Read the model definition and answer for the solid it produces. Units are mm, in the model's axes. A direction names the side the tool comes from. Round coordinates to 2 decimals unless told otherwise and drop trailing zeros. Write each loop counter-clockwise with the first axis right and the second up, starting at its lowest first coordinate (ties: lowest second). Pieces come first, ordered by that corner, then holes.
from build123d import *

# Parameters (mm, degrees)
BOSS_EXTRUDE1_DEPTH = 46.736
SKETCH3_W           = 38.481
SKETCH3_H           = 38.481
BOSS_EXTRUDE2_DEPTH = 17.526
SKETCH_D_R          = 7.9375
BOSS_EXTRUDE3_DEPTH = 38.1
CUT_EXTRUDE1_DEPTH  = 35.56
FILLET1_R           = 6.35
FILLET2_R           = 1.27
KEYWAY_START        = 5.1943
KEYWAY_DEPTH        = 33.9057
CHAMFER1_SIZE       = 0.381
SKETCH7_R           = 7.9375
CUT_EXTRUDE3_DEPTH  = 103.362


with BuildPart() as part:
    # L,M → Boss-Extrude1 (new body)
    with BuildSketch(Plane.XY):
        Polygon((-44.45, 31.75), (44.45, 31.75), (44.45, 90.644463274), (36.576, 98.518463274), (36.576, 130.081536726), (14.257536726, 152.4), (-14.257536726, 152.4), (-36.576, 130.081536726), (-36.576, 98.518463274), (-44.45, 90.644463274), align=None)
    extrude(amount=BOSS_EXTRUDE1_DEPTH)

    # Sketch3 → Boss-Extrude2 (add)
    with BuildSketch(Plane.XY.offset(46.736)):
        with Locations((0, 114.3)):
            Rectangle(SKETCH3_W, SKETCH3_H)
    extrude(amount=BOSS_EXTRUDE2_DEPTH)

    # D → Boss-Extrude3 (add)
    with BuildSketch(Plane.XY.offset(64.262)):
        with Locations((0, 114.3)):
            Circle(SKETCH_D_R)
    extrude(amount=BOSS_EXTRUDE3_DEPTH)

    # Sketch5 → Cut-Extrude1 (cut)
    with BuildSketch(Plane.XY.offset(46.736)):
        Polygon((44.45, 54.068463274), (22.131536726, 31.75), (44.45, 31.75), align=None)
        Polygon((-44.45, 31.75), (-44.45, 54.068463274), (-22.131536726, 31.75), align=None)
    extrude(amount=-CUT_EXTRUDE1_DEPTH, mode=Mode.SUBTRACT)

    # Fillet1
    fillet1_edges = [part.edges().sort_by_distance(p)[0] for p in [
        (-19.2405, 133.5405, 55.499),
        (-19.2405, 95.0595, 55.499),
        (19.2405, 95.0595, 55.499),
        (19.2405, 133.5405, 55.499),
    ]]
    fillet(fillet1_edges, radius=FILLET1_R)

    # Fillet2
    fillet2_edges = [part.edges().sort_by_distance(p)[0] for p in [
        (44.45, 72.356463274, 46.736),
        (33.290768363, 42.909231637, 46.736),
        (40.513, 94.581463274, 46.736),
        (36.576, 114.3, 46.736),
        (25.416768363, 141.240768363, 46.736),
        (0, 31.75, 46.736),
        (0, 152.4, 46.736),
        (-25.416768363, 141.240768363, 46.736),
        (-36.576, 114.3, 46.736),
        (-40.513, 94.581463274, 46.736),
        (-44.45, 72.356463274, 46.736),
        (-33.290768363, 42.909231637, 46.736),
        (0, 95.0595, 46.736),
        (-19.2405, 114.3, 46.736),
        (19.2405, 114.3, 46.736),
        (0, 133.5405, 46.736),
        (-17.380628061, 96.919371939, 46.736),
        (17.380628061, 96.919371939, 46.736),
        (-17.380628061, 131.680628061, 46.736),
        (17.380628061, 131.680628061, 46.736),
    ]]
    fillet(fillet2_edges, radius=FILLET2_R)

    # Sketch6 → Keyway (cut, through all)
    with BuildSketch(Plane(origin=(0, 114.3, 0), x_dir=(-1, 0, 0), z_dir=(0, 1, 0)).offset(KEYWAY_START)):
        with BuildLine():
            Line((2.3876, 102.362), (2.3876, 69.342))
            ThreePointArc((2.3876, 69.342), (0, 66.9544), (-2.3876, 69.342))
            Line((-2.3876, 69.342), (-2.3876, 102.362))
            ThreePointArc((-2.3876, 102.362), (0, 104.7496), (2.3876, 102.362))
        make_face()
    extrude(amount=KEYWAY_DEPTH, mode=Mode.SUBTRACT)

    # Chamfer1
    chamfer1_edges = [part.edges().sort_by_distance(p)[0] for p in [
        (-4.693204196, 107.898614164, 102.362),
    ]]
    chamfer(chamfer1_edges, length=CHAMFER1_SIZE)

    # Sketch7 → Cut-Extrude3 (cut, through all)
    with BuildSketch(Plane(origin=(0, 0, 0), x_dir=(-1, 0, 0), z_dir=(0, 0, -1))):
        with Locations((0, 63.5)):
            Circle(SKETCH7_R)
    extrude(amount=-CUT_EXTRUDE3_DEPTH, mode=Mode.SUBTRACT)


solid = part.part
Q1. Straight lines are drawn through the part: probe 1 along X at (y, z) = (63, 27); probe 2 along Y at (x, z) = (0, 27); probe 3 along Z at (x, y) = (19, 66). For each, find the intervals that lie inside material, in ascending order.
Verdict:
probe 1: x = -44.45 to -7.92, 7.92 to 44.45
probe 2: y = 31.75 to 55.56, 71.44 to 152.4
probe 3: z = 0 to 46.74
Q2. Determine the mould class of faces 1 (the cylindrical face through (1.72, 55.75, 23.04)), 2 (the cylindrical face through (-40.115, 94.44, 46.374)) for opening direction Z: pulls with the +Z half, pulls with the -Z half, needs draft (parallel to the pull), parting line crosses it, or undercut.
Verdict:
face 1: needs draft
face 2: pulls with the +Z half
Q3. Which of the six approach directions +Z, -Z, +X, -X, +Y, -Y give full straight-line access (tool end or side, diameter ignored) to faces 3 (the cylindrical face through (-1.72, 106.55, 82.86)), 4 (the flat face through (0, 133.54, 56)), 5 (the cylindrical face through (-17.43, 131.63, 56.25)), 6 (the flat face through (-19.24, 114, 56)), 7 (the flat face through (19.24, 114, 56))?
Verdict:
face 3: +Z
face 4: +Z, +X, -X, +Y
face 5: +Z, -X, +Y
face 6: +Z, -X, +Y, -Y
face 7: +Z, +X, +Y, -Y
Q4. Section A-A (y = 63.5) is taken. Determine the outline of the cut face in (x, z), then the cut area to 3 significant figures.
Verdict:
outline: (-44.45, 0) - (-7.94, 0) - (-7.94, 46.74) - (-43.18, 46.74) arc R1.27 ccw to (-44.45, 45.47) - close; (7.94, 0) - (44.45, 0) - (44.45, 45.47) arc R1.27 ccw to (43.18, 46.74) - (7.94, 46.74) - close
area: 3,410 mm2
Q5. Section D-D (y = 87.5) is taken. Determine the outline of the cut face in (x, z), then the cut area to 3 significant figures.
Verdict:
outline: (-44.45, 0) - (44.45, 0) - (44.45, 45.47) arc R1.27 ccw to (43.18, 46.74) - (-43.18, 46.74) arc R1.27 ccw to (-44.45, 45.47) - close
area: 4,150 mm2
Q6. Section C-C (x = 0) is taken. Determine the outline of the cut face in (y, z).
Verdict:
outline: (31.75, 0) - (55.56, 0) - (55.56, 46.74) - (33.02, 46.74) arc R1.27 ccw to (31.75, 45.47) - close; (71.44, 0) - (152.4, 0) - (152.4, 45.47) arc R1.27 ccw to (151.13, 46.74) - (134.81, 46.74) arc R1.27 cw to (133.54, 48.01) - (133.54, 64.26) - (122.24, 64.26) - (122.24, 66.95) - (119.49, 66.95) - (119.49, 102.36) - (106.74, 102.36) - (106.36, 101.98) - (106.36, 64.26) - (95.06, 64.26) - (95.06, 48.01) arc R1.27 cw to (93.79, 46.74) - (71.44, 46.74) - close
Q7. Flat-ended cylindrical pins translate along their axes: pin 1 Ø12 at (y, z) = (107.5, 26.5) entering from +X; pin 2 Ø8 at (y, z) = (120, 60) entering from -X; pin 3 Ø8 at (x, z) = (-6, 58.5) entering from +Y; pin 4 Ø9.5 at (x, y) = (0, 63.5) entering from -Z. Find the tip coordinate at first contact, or state that the pin passes through.
Verdict:
pin 1: stops at x = 36.58
pin 2: stops at x = -19.24
pin 3: stops at y = 133.54
pin 4: passes through
